Check sheet for the modelled part. Datum: model origin and axes. Units: mm. Face numbers are marked on the shaded views. A direction names the side the tool comes from. Give positions to 0.01 mm unless a question says otherwise; leave off trailing zeros. Loops run counter-clockwise (first coordinate to the right, second up) from the corner with the lowest first, then second, coordinate; pieces in that order, holes last. Notation, with made-up numbers: (-22.5, -30.75) - (22.5, -30.75) arc R29 cw to (22.5, 4.25) - close; hole circle Ø1 at (71.25, -20.5). An arc over 180 degrees is marked (long way). Answer in a Markdown table with one row per item. Add a question column.
(1) Sectioned sample at C-C on y = 13. Enter the section's corners in (x, z), then the cut area to 3 significant figures.
(2) Sectioned sample at B-B on x = 0. Enter the section's corners in (y, z).
(3) Go/stop test with flat-tipped pins: P1, Ø3, axis at y = -8, z = -5.5, coming from the +X side; P2, Ø0.8, axis at y = -1.5, z = 1.5, coming from the +X side; P3, Ø4, axis at y = -5, z = -6.5, coming from the -X side. Record where each tip stops, or that it passes through.
(4) Thickness scan on L1, parallel to X at y = 22, z = -4.75; L2, parallel to X at y = 10.5, z = -2.75; L3, parallel to X at y = -5.5, z = -6.25. Record the ranges inside material, lowest first.
(5) Sectioned sample at A-A on y = 3.5. Enter the section's corners in (x, z).
(6) Set-up check for the marked faces 4, 5, 6 and 7: record each of +Z, -Z, +X, -X, +Y, -Y from which the full face is reachable in a straight line by a thin tool's end or side.
(7) Sectioned sample at D-D on y = -10.5. Enter the section's corners in (x, z), then the cut area to 3 significant figures.
(8) Draft check along X on the marked faces 1, 2 and 3. Enter one of: released by +X, released by -X, zero draft, split by the parting line, or undercut.
from build123d import *

# Parameters (mm, degrees)
EXTRUDE_THIN1_DEPTH = 9
BOSS_EXTRUDE1_START = 2.5
BOSS_EXTRUDE1_DEPTH = 2.5
SKETCH7_W           = 10.4
SKETCH7_H           = 2
CUT_EXTRUDE2_DEPTH  = 9
FILLET1_R           = 2
FILLET2_R           = 1
FILLET3_R           = 1


with BuildPart() as part:
    # Sketch4 → Extrude-Thin1 (new body)
    with BuildSketch(Plane.XY):
        with BuildLine():
            ThreePointArc((-27.9, 10.565509926), (-22.336413862, 5.001923789), (-20.3, -2.598076211))
            Line((-20.3, -2.598076211), (-20.3, -13))
            ThreePointArc((-20.3, -13), (-20.132058957, -13.759199288), (-19.659573823, -14.37673111))
            Line((-19.659573823, -14.37673111), (-11.593677676, -6.310834964))
            ThreePointArc((-11.593677676, -6.310834964), (-13.132911027, 1.329153101), (-10.094117647, 8.505809128))
            ThreePointArc((-10.094117647, 8.505809128), (-6.461802118, 14.774561158), (-5.2, 21.9089023))
            Line((-5.2, 21.9089023), (5.2, 21.9089023))
            ThreePointArc((5.2, 21.9089023), (6.461802118, 14.774561158), (10.094117647, 8.505809128))
            ThreePointArc((10.094117647, 8.505809128), (13.132911027, 1.329153101), (11.593677676, -6.310834964))
            Line((11.593677676, -6.310834964), (19.659573823, -14.37673111))
            ThreePointArc((19.659573823, -14.37673111), (20.132058957, -13.759199288), (20.3, -13))
            Line((20.3, -13), (20.3, -2.598076211))
            ThreePointArc((20.3, -2.598076211), (22.336413862, 5.001923789), (27.9, 10.565509926))
            Line((27.9, 10.565509926), (26.9, 12.297560734))
            ThreePointArc((26.9, 12.297560734), (20.604363055, 6.001923789), (18.3, -2.598076211))
            Line((18.3, -2.598076211), (18.3, -10.188730163))
            Line((18.3, -10.188730163), (14.009117998, -5.897848161))
            ThreePointArc((14.009117998, -5.897848161), (15.027346247, 2.28448348), (11.623529412, 9.794568087))
            ThreePointArc((11.623529412, 9.794568087), (8.022061411, 16.410382128), (7.306685687, 23.9089023))
            Line((7.306685687, 23.9089023), (-7.306685687, 23.9089023))
            ThreePointArc((-7.306685687, 23.9089023), (-8.022061411, 16.410382128), (-11.623529412, 9.794568087))
            ThreePointArc((-11.623529412, 9.794568087), (-15.027346247, 2.28448348), (-14.009117998, -5.897848161))
            Line((-14.009117998, -5.897848161), (-18.3, -10.188730163))
            Line((-18.3, -10.188730163), (-18.3, -2.598076211))
            ThreePointArc((-18.3, -2.598076211), (-20.604363055, 6.001923789), (-26.9, 12.297560734))
            Line((-26.9, 12.297560734), (-27.9, 10.565509926))
        make_face()
    extrude(amount=-EXTRUDE_THIN1_DEPTH)

    # Sketch5 → Boss-Extrude1 (add)
    with BuildSketch(Plane.XY.offset(BOSS_EXTRUDE1_START)):
        with BuildLine():
            Line((-26.9, 12.297560734), (-7.306685687, 23.9089023))
            ThreePointArc((-7.306685687, 23.9089023), (-8.022061411, 16.410382128), (-11.623529412, 9.794568087))
            ThreePointArc((-11.623529412, 9.794568087), (-15.027346247, 2.28448348), (-14.009117998, -5.897848161))
            Line((-14.009117998, -5.897848161), (-18.3, -10.188730163))
            Line((-18.3, -10.188730163), (-18.3, -2.598076211))
            ThreePointArc((-18.3, -2.598076211), (-20.604363055, 6.001923789), (-26.9, 12.297560734))
        make_face()
        with BuildLine():
            ThreePointArc((-18.3, -2.598076211), (-20.604363055, 6.001923789), (-26.9, 12.297560734))
            Line((-26.9, 12.297560734), (-27.9, 10.565509926))
            ThreePointArc((-27.9, 10.565509926), (-22.336413862, 5.001923789), (-20.3, -2.598076211))
            Line((-20.3, -2.598076211), (-20.3, -13))
            ThreePointArc((-20.3, -13), (-20.132058957, -13.759199288), (-19.659573823, -14.37673111))
            Line((-19.659573823, -14.37673111), (-19.555634919, -14.272792206))
            Line((-19.555634919, -14.272792206), (-11.593677676, -6.310834964))
            ThreePointArc((-11.593677676, -6.310834964), (-13.132911027, 1.329153101), (-10.094117647, 8.505809128))
            ThreePointArc((-10.094117647, 8.505809128), (-6.461802118, 14.774561158), (-5.2, 21.9089023))
            Line((-5.2, 21.9089023), (5.2, 21.9089023))
            ThreePointArc((5.2, 21.9089023), (6.461802118, 14.774561158), (10.094117647, 8.505809128))
            ThreePointArc((10.094117647, 8.505809128), (13.132911027, 1.329153101), (11.593677676, -6.310834964))
            Line((11.593677676, -6.310834964), (19.555634919, -14.272792206))
            Line((19.555634919, -14.272792206), (19.659573823, -14.37673111))
            ThreePointArc((19.659573823, -14.37673111), (20.132058957, -13.759199288), (20.3, -13))
            Line((20.3, -13), (20.3, -2.598076211))
            ThreePointArc((20.3, -2.598076211), (22.336413862, 5.001923789), (27.9, 10.565509926))
            Line((27.9, 10.565509926), (26.9, 12.297560734))
            ThreePointArc((26.9, 12.297560734), (20.604363055, 6.001923789), (18.3, -2.598076211))
            Line((18.3, -2.598076211), (18.3, -10.188730163))
            Line((18.3, -10.188730163), (14.009117998, -5.897848161))
            ThreePointArc((14.009117998, -5.897848161), (15.027346247, 2.28448348), (11.623529412, 9.794568087))
            ThreePointArc((11.623529412, 9.794568087), (8.022061411, 16.410382128), (7.306685687, 23.9089023))
            Line((7.306685687, 23.9089023), (-7.306685687, 23.9089023))
            ThreePointArc((-7.306685687, 23.9089023), (-8.022061411, 16.410382128), (-11.623529412, 9.794568087))
            ThreePointArc((-11.623529412, 9.794568087), (-15.027346247, 2.28448348), (-14.009117998, -5.897848161))
            Line((-14.009117998, -5.897848161), (-18.3, -10.188730163))
            Line((-18.3, -10.188730163), (-18.3, -2.598076211))
        make_face()
        with BuildLine():
            Line((7.306685687, 23.9089023), (26.9, 12.297560734))
            ThreePointArc((26.9, 12.297560734), (20.604363055, 6.001923789), (18.3, -2.598076211))
            Line((18.3, -2.598076211), (18.3, -10.188730163))
            Line((18.3, -10.188730163), (14.009117998, -5.897848161))
            ThreePointArc((14.009117998, -5.897848161), (15.027346247, 2.28448348), (11.623529412, 9.794568087))
            ThreePointArc((11.623529412, 9.794568087), (8.022061411, 16.410382128), (7.306685687, 23.9089023))
        make_face()
        with BuildLine():
            ThreePointArc((-10.094117647, 8.505809128), (-13.132911027, 1.329153101), (-11.593677676, -6.310834964))
            Line((-11.593677676, -6.310834964), (-10.727207794, -5.444365081))
            ThreePointArc((-10.727207794, -5.444365081), (-10.337016841, -4.860403054), (-10.2, -4.171572875))
            Line((-10.2, -4.171572875), (-10.2, 0))
            ThreePointArc((-10.2, 0), (0, 10.2), (10.2, 0))
            Line((10.2, 0), (10.2, -4.171572875))
            ThreePointArc((10.2, -4.171572875), (10.337016841, -4.860403054), (10.727207794, -5.444365081))
            Line((10.727207794, -5.444365081), (11.593677676, -6.310834964))
            ThreePointArc((11.593677676, -6.310834964), (13.132911027, 1.329153101), (10.094117647, 8.505809128))
            ThreePointArc((10.094117647, 8.505809128), (6.461802118, 14.774561158), (5.2, 21.9089023))
            Line((5.2, 21.9089023), (-5.2, 21.9089023))
            ThreePointArc((-5.2, 21.9089023), (-6.461802118, 14.774561158), (-10.094117647, 8.505809128))
        make_face()
    extrude(amount=-BOSS_EXTRUDE1_DEPTH)

    # Sketch7 → Cut-Extrude2 (cut)
    with BuildSketch(Plane.XY.offset(-9)):
        with Locations((0, 22.9089023)):
            Rectangle(SKETCH7_W, SKETCH7_H)
    extrude(amount=CUT_EXTRUDE2_DEPTH, mode=Mode.SUBTRACT)

    # Fillet1
    fillet1_edges = [part.edges().sort_by_distance(p)[0] for p in [
        (27.9, 10.565509926, -3.25),
        (-27.9, 10.565509926, -3.25),
    ]]
    fillet(fillet1_edges, radius=FILLET1_R)

    # Fillet2
    # the kernel refuses this fillet: 1 mm, written as the material it takes off along each edge
    with BuildSketch(Plane(origin=(19.659573823, -14.37673111, -13.714649626), x_dir=(0.33959372810271005, 0.9405722193608009, 0), z_dir=(0, 0, 1))) as fillet2_piece_1:
        with BuildLine():
            CenterArc((1.546266122, 0.940572219), FILLET2_R, 154.852123731, 135)
            Line((0.6410521, 1.365528186), (0.550530698, 1.408023783))
            Line((0.550530698, 1.408023783), (-0.090521402, 0.042495597))
            Line((-0.090521402, 0.042495597), (-0.050062835, -0.086566232))
            ThreePointArc((-0.050062835, -0.086566232), (1.546359122, -0.228895043), (1.919819223, -0.094057222))
            Line((1.919819223, -0.094057222), (1.885859851, 0))
        make_face()
    extrude(amount=20.929299253, mode=Mode.SUBTRACT)
    with BuildSketch(Plane(origin=(-19.659573823, -14.37673111, -13.714649626), x_dir=(-0.3395937281027359, 0.9405722193607915, 0), z_dir=(0, 0, 1))) as fillet2_piece_2:
        with BuildLine():
            CenterArc((1.546266122, -0.940572219), FILLET2_R, 70.147876269, 135)
            Line((0.6410521, -1.365528186), (0.550530698, -1.408023783))
            Line((0.550530698, -1.408023783), (-0.090521402, -0.042495597))
            Line((-0.090521402, -0.042495597), (-0.050062835, 0.086566232))
            ThreePointArc((-0.050062835, 0.086566232), (1.546359122, 0.228895043), (1.919819223, 0.094057222))
            Line((1.919819223, 0.094057222), (1.885859851, 0))
        make_face()
    extrude(amount=20.929299253, mode=Mode.SUBTRACT)

    # Fillet3
    fillet3_edges = [part.edges().sort_by_distance(p)[0] for p in [
        (-5.2, 23.9089023, -4.5),
        (5.2, 23.9089023, -4.5),
        (-18.3, -10.188730163, -4.5),
        (-14.009117998, -5.897848161, -4.5),
        (14.009117998, -5.897848161, -4.5),
        (18.3, -10.188730163, -4.5),
        (11.593677676, -6.310834964, -4.5),
        (-11.593677676, -6.310834964, -4.5),
    ]]
    fillet(fillet3_edges, radius=FILLET3_R)


solid = part.part
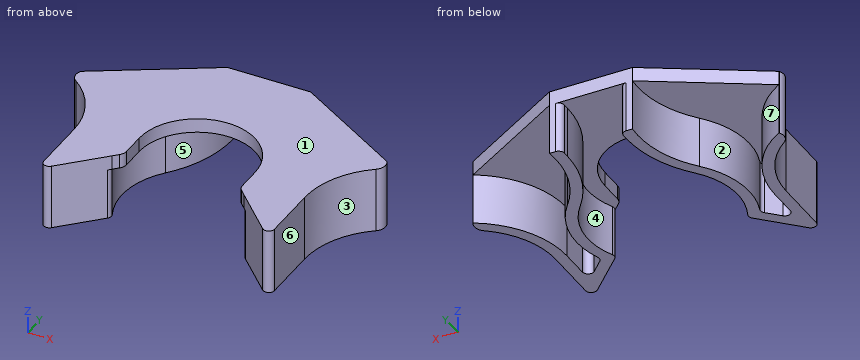
Reply:
| question | item | result |
|---|---|---|
| 1 | outline | (-25.71, 0) - (-9.44, 0) - (-9.44, -9) - (-7.2, -9) - (-7.2, 0) - (7.2, 0) - (7.2, -9) - (9.44, -9) - (9.44, 0) - (25.71, 0) - (25.71, 2.5) - (-25.71, 2.5) - close |
| 1 | area | 169 mm^2 |
| 2 | outline | (10.2, 0) - (23.91, 0) - (23.91, 2.5) - (10.2, 2.5) - close |
| 3 | P1 | x = 20.3 |
| 3 | P2 | x = 20.37 |
| 3 | P3 | x = -20.3 |
| 4 | L1 | -7.2 to -5.2, 5.2 to 7.2 |
| 4 | L2 | -27.1 to -24.35, -11.06 to -8.61, 8.61 to 11.06, 24.35 to 27.1 |
| 4 | L3 | -20.3 to -18.3, -14.19 to -12, 12 to 14.19, 18.3 to 20.3 |
| 5 | outline | (-21.58, -9) - (-19.42, -9) - (-19.42, 0) - (-14.79, 0) - (-14.79, -9) - (-12.73, -9) - (-12.73, 0) - (-9.58, 0) - (-9.58, 2.5) - (-21.58, 2.5) - close; (9.58, 0) - (12.73, 0) - (12.73, -9) - (14.79, -9) - (14.79, 0) - (19.42, 0) - (19.42, -9) - (21.58, -9) - (21.58, 2.5) - (9.58, 2.5) - close |
| 6 | face 4 | -Z |
| 6 | face 5 | -Z, -Y |
| 6 | face 6 | +Z, -Z, +X, -Y |
| 6 | face 7 | -Z, +Y |
| 7 | outline | (-20.3, -9) - (-15.78, -9) - (-15.78, 2.5) - (-20.3, 2.5) - close; (15.78, -9) - (20.3, -9) - (20.3, 2.5) - (15.78, 2.5) - close |
| 7 | area | 104 mm^2 |
| 8 | face 1 | zero draft |
| 8 | face 2 | undercut |
| 8 | face 3 | released by +X |
